from build123d import *

# Parameters (mm, degrees)
BOSS_EXTRUDE2_DEPTH = 49
CUT_EXTRUDE1_REACH  = 113.521
SKETCH4_R           = 1.25
SKETCH4_R_2         = 8
CUT_EXTRUDE3_REACH  = 113.521
FILLET2_R           = 1


with BuildPart() as part:
    # Sketch3 → Boss-Extrude2 (new body)
    with BuildSketch(Plane(origin=(0, 0, 0), x_dir=(0, 0, -1), z_dir=(1, 0, 0))):
        Polygon((0, 0), (2, 0), (2, -42), (88, -42), (88, -32), (90, -32), (90, -44), (0, -44), align=None)
    extrude(amount=BOSS_EXTRUDE2_DEPTH)

    # Sketch4 → Cut-Extrude1 (cut, up to next)
    with BuildSketch(Plane.XY, mode=Mode.PRIVATE) as cut_extrude1_sk1:
        with Locations((24.5, -34)):
            Circle(SKETCH4_R)
    cut_extrude1_tool1 = extrude(cut_extrude1_sk1.sketch, amount=-CUT_EXTRUDE1_REACH, mode=Mode.PRIVATE) & part.part
    # Sketch4 → Cut-Extrude1 (cut, up to next)
    with BuildSketch(Plane.XY, mode=Mode.PRIVATE) as cut_extrude1_sk2:
        with Locations((14.107695155, -16)):
            Circle(SKETCH4_R)
    cut_extrude1_tool2 = extrude(cut_extrude1_sk2.sketch, amount=-CUT_EXTRUDE1_REACH, mode=Mode.PRIVATE) & part.part
    # Sketch4 → Cut-Extrude1 (cut, up to next)
    with BuildSketch(Plane.XY, mode=Mode.PRIVATE) as cut_extrude1_sk3:
        with Locations((34.892304845, -16)):
            Circle(SKETCH4_R)
    cut_extrude1_tool3 = extrude(cut_extrude1_sk3.sketch, amount=-CUT_EXTRUDE1_REACH, mode=Mode.PRIVATE) & part.part
    # Sketch4 → Cut-Extrude1 (cut, up to next)
    with BuildSketch(Plane.XY, mode=Mode.PRIVATE) as cut_extrude1_sk4:
        with Locations((24.5, -22)):
            Circle(SKETCH4_R_2)
    cut_extrude1_tool4 = extrude(cut_extrude1_sk4.sketch, amount=-CUT_EXTRUDE1_REACH, mode=Mode.PRIVATE) & part.part
    add(cut_extrude1_tool1.solids().sort_by_distance((24.5, -34, 0))[0], mode=Mode.SUBTRACT)
    add(cut_extrude1_tool2.solids().sort_by_distance((14.107695, -16, 0))[0], mode=Mode.SUBTRACT)
    add(cut_extrude1_tool3.solids().sort_by_distance((34.892305, -16, 0))[0], mode=Mode.SUBTRACT)
    add(cut_extrude1_tool4.solids().sort_by_distance((24.5, -22, 0))[0], mode=Mode.SUBTRACT)

    # Sketch5 → Cut-Extrude3 (cut, up to next)
    with BuildSketch(Plane.XZ.offset(44), mode=Mode.PRIVATE) as cut_extrude3_sk1:
        with BuildLine():
            Line((41, -17), (41, -33))
            ThreePointArc((41, -33), (43, -35), (45, -33))
            Line((45, -33), (45, -17))
            ThreePointArc((45, -17), (43, -15), (41, -17))
        make_face()
    cut_extrude3_tool1 = extrude(cut_extrude3_sk1.sketch, amount=-CUT_EXTRUDE3_REACH, mode=Mode.PRIVATE) & part.part
    # Sketch5 → Cut-Extrude3 (cut, up to next)
    with BuildSketch(Plane.XZ.offset(44), mode=Mode.PRIVATE) as cut_extrude3_sk2:
        with BuildLine():
            Line((45, -73), (45, -57))
            ThreePointArc((45, -57), (43, -55), (41, -57))
            Line((41, -57), (41, -73))
            ThreePointArc((41, -73), (43, -75), (45, -73))
        make_face()
    cut_extrude3_tool2 = extrude(cut_extrude3_sk2.sketch, amount=-CUT_EXTRUDE3_REACH, mode=Mode.PRIVATE) & part.part
    # Sketch5 → Cut-Extrude3 (cut, up to next)
    with BuildSketch(Plane.XZ.offset(44), mode=Mode.PRIVATE) as cut_extrude3_sk3:
        with BuildLine():
            Line((8, -73), (8, -57))
            ThreePointArc((8, -57), (6, -55), (4, -57))
            Line((4, -57), (4, -73))
            ThreePointArc((4, -73), (6, -75), (8, -73))
        make_face()
    cut_extrude3_tool3 = extrude(cut_extrude3_sk3.sketch, amount=-CUT_EXTRUDE3_REACH, mode=Mode.PRIVATE) & part.part
    # Sketch5 → Cut-Extrude3 (cut, up to next)
    with BuildSketch(Plane.XZ.offset(44), mode=Mode.PRIVATE) as cut_extrude3_sk4:
        with BuildLine():
            Line((4, -17), (4, -33))
            ThreePointArc((4, -33), (6, -35), (8, -33))
            Line((8, -33), (8, -17))
            ThreePointArc((8, -17), (6, -15), (4, -17))
        make_face()
    cut_extrude3_tool4 = extrude(cut_extrude3_sk4.sketch, amount=-CUT_EXTRUDE3_REACH, mode=Mode.PRIVATE) & part.part
    add(cut_extrude3_tool1.solids().sort_by_distance((43, -44, -25))[0], mode=Mode.SUBTRACT)
    add(cut_extrude3_tool2.solids().sort_by_distance((43, -44, -65))[0], mode=Mode.SUBTRACT)
    add(cut_extrude3_tool3.solids().sort_by_distance((6, -44, -65))[0], mode=Mode.SUBTRACT)
    add(cut_extrude3_tool4.solids().sort_by_distance((6, -44, -25))[0], mode=Mode.SUBTRACT)

    # Fillet2
    fillet2_edges = [part.edges().sort_by_distance(p)[0] for p in [
        (0, 0, -1),
        (24.5, -44, 0),
        (24.5, -44, -90),
        (49, -32, -89),
        (49, 0, -1),
        (0, -32, -89),
    ]]
    fillet(fillet2_edges, radius=FILLET2_R)


solid = part.part
Geometry: final body of the model. Coordinates: model frame, mm. A direction names the side the tool comes from. Give positions to 0.01 mm unless a question says otherwise; leave off trailing zeros. Write each loop counter-clockwise with the first axis right and the second up, starting at its lowest first coordinate (ties: lowest second). Pieces come first, ordered by that corner, then holes. Notation, with made-up numbers: M -1.5,75.5 L 47.5,75.5 A29 ccw 47.5,114.5 Z; hole C -40,-35 d7. An arc over 180 degrees is marked long. Answer in a Markdown table with one row per item. Add a question column.
(1) Section B-B on z = -63. Return loops of the section in (x, y).
(2) Section C-C on x = 43. Return loops of the section in (y, z), and give its area (3 significant figures).
(3) Mould query, pull axis Z, two halves, no side actions, for faces 6 (the cylindrical face through (18.151, -26.868, -0.986)), 7 (the flat face through (24, -31, 0)), 8 (the flat face through (18.7, -16, -2)). Classes: +Z half, -Z half, draft (parallel to the pull), parting line (faces both ways), or undercut.
(4) Reachability of faces 1 (the cylindrical face through (25.655, -34.479, -0.986)), 2 (the flat face through (24, -37, -88)), 3 (the cylindrical face through (43, -43, -15)), 4 (the flat face through (24, -44, -46)), 5 (the cylindrical face through (14.78, -14.946, -0.986)) from +Z, -Z, +X, -X, +Y, -Y: full face, straight path, thin tool, end or side. Return the list, or none.
(5) First-contact query: pin 1 (1 mm diameter, centred on x = 35, z = -88.5, fed in from +Y); pin 2 (8 mm diameter, centred on x = 13, z = -46, fed in from +Y); pin 3 (12 mm diameter, centred on x = 5.5, y = -6.5, fed in from -Z). Flat tips, straight axial feed; report the tip coordinate or a pass-through.
(6) Ray query, line 1 (Y direction, x = 24.5, z = -1.2); line 2 (Z direction, x = 9, y = -41); line 3 (Y direction, x = 34.5, z = -81.5). Return the intervals inside material, ascending.
(7) Section D-D on y = -16. Return loops of the section in (x, z).
(8) Section A-A on y = -39. Return loops of the section in (x, z).
Result set:
| question | item | result |
|---|---|---|
| 1 | outline | M 0,-44 L 4,-44 L 4,-42 L 0,-42 Z; M 8,-44 L 41,-44 L 41,-42 L 8,-42 Z; M 45,-44 L 49,-44 L 49,-42 L 45,-42 Z |
| 2 | outline | M -44,-89 A1 ccw -43,-90 L -32,-90 L -32,-88 L -42,-88 L -42,-75 L -44,-75 Z; M -44,-55 L -42,-55 L -42,-35 L -44,-35 Z; M -44,-15 L -42,-15 L -42,-2 L 0,-2 L 0,0 L -43,0 A1 ccw -44,-1 Z |
| 2 | area | 204 mm^2 |
| 3 | face 6 | draft |
| 3 | face 7 | +Z half |
| 3 | face 8 | undercut |
| 4 | face 1 | +Z |
| 4 | face 2 | +X, -X, +Y |
| 4 | face 3 | +Y, -Y |
| 4 | face 4 | +Z, -Z, +X, -X, -Y |
| 4 | face 5 | +Z, -Z |
| 5 | pin 1 | stops at y = -32 |
| 5 | pin 2 | stops at y = -42 |
| 5 | pin 3 | stops at z = -2 |
| 6 | line 1 | y = -44 to -35.25, -32.75 to -30, -14 to 0 |
| 6 | line 2 | z = -90 to -88, -2 to 0 |
| 6 | line 3 | y = -44 to -42 |
| 7 | outline | M 0,-2 L 12.86,-2 L 12.86,0 L 0,0 Z; M 15.36,-2 L 19.21,-2 L 19.21,0 L 15.36,0 Z; M 29.79,-2 L 33.64,-2 L 33.64,0 L 29.79,0 Z; M 36.14,-2 L 49,-2 L 49,0 L 36.14,0 Z |
| 8 | outline | M 0,-90 L 49,-90 L 49,-88 L 0,-88 Z; M 0,-2 L 49,-2 L 49,0 L 0,0 Z |
